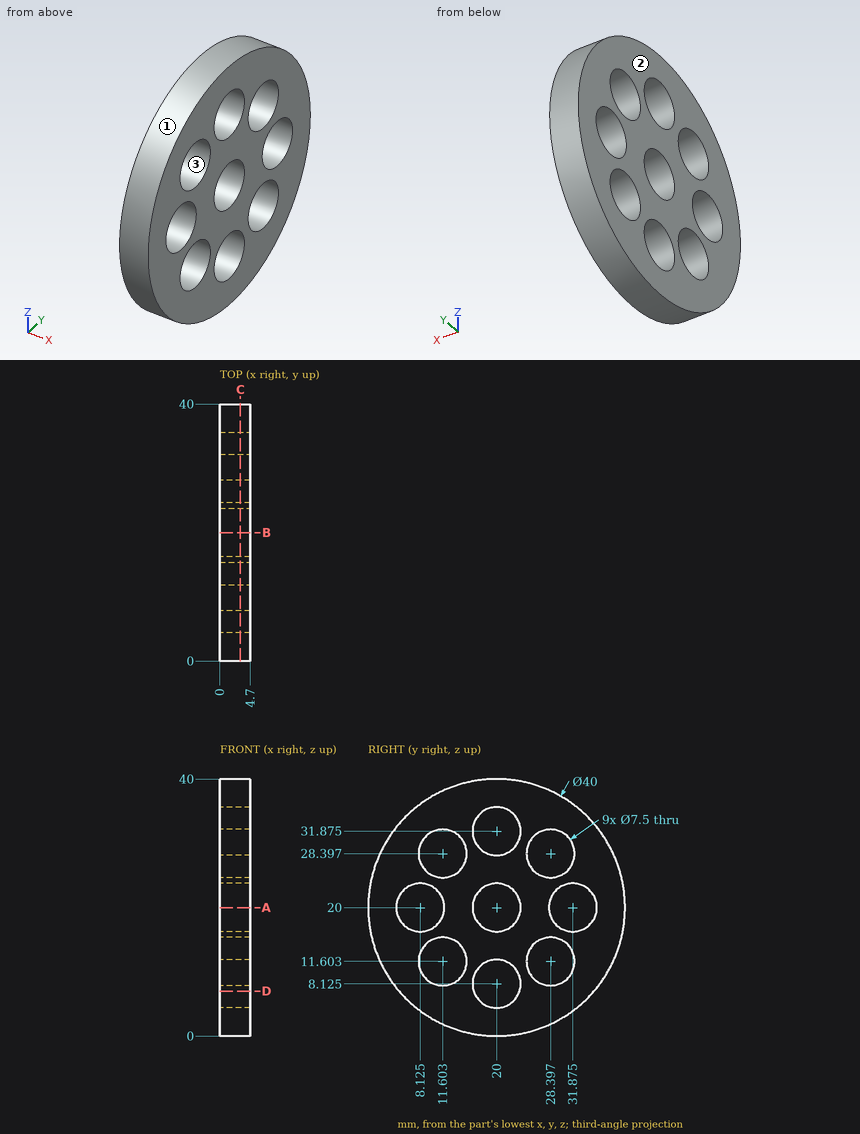
Input: dimensioned drawing with shaded views. Units: mm. Origin: part minimum x, y, z. Give positions to 0.01 mm unless a question says otherwise; leave off trailing zeros. Write each loop counter-clockwise with the first axis right and the second up, starting at its lowest first coordinate (ties: lowest second). Pieces come first, ordered by that corner, then holes. Notation, with made-up numbers: (-13.5, -23) - (9.5, -23) arc R17 cw to (9.5, -2) - close; hole circle Ø9 at (17.5, 7.25). An arc over 180 degrees is marked (long way). Write item = value, one per line. Start each with the question number.
1) Pin query (flat end, axial travel): pin 1 (1 mm diameter, centred on x = 1, y = 6, fed in from -Z); pin 2 (2 mm diameter, centred on x = 2, z = 27.5, fed in from -Y). Return the tip coordinate at first contact, or that it passes through.
2) Cut plane D-D (z = 7). Return loops of the section in (x, y), and give its area (3 significant figures).
3) Cut plane A-A (z = 20). Return loops of the section in (x, y) (3 decimals).
4) Cut plane C-C (x = 3.2). Give the number of separate pieces and of enclosed holes in the cut face, and give its area (3 significant figures).
5) Draft query along Y for the marked faces 1, 2 and 3. Return one class per face: pulls with the +Y half, pulls with the -Y half, needs draft (parallel to the pull), parting line crosses it, or undercut.
6) Material intervals for L1, parallel to Z at x = 2.1, y = 20 (3 decimals); L2, parallel to Z at x = 2.7, y = 22; L3, parallel to Y at x = 0.25, z = 28, sorted ascending. Write a range as [from, to].
Answers follow:
q1.pin_1 = 5.24
q1.pin_2 = 1.09
q2.outline = (0, 4.8) - (4.7, 4.8) - (4.7, 16.42) - (0, 16.42) - close; (0, 23.58) - (4.7, 23.58) - (4.7, 35.2) - (0, 35.2) - close
q2.area = 109 mm^2
q3.outline = (0, 0) - (4.7, 0) - (4.7, 4.375) - (0, 4.375) - close; (0, 11.875) - (4.7, 11.875) - (4.7, 16.25) - (0, 16.25) - close; (0, 23.75) - (4.7, 23.75) - (4.7, 28.125) - (0, 28.125) - close; (0, 35.625) - (4.7, 35.625) - (4.7, 40) - (0, 40) - close
q4.separate_pieces = 1
q4.enclosed_holes = 9
q4.area = 859 mm^2
q5.face_1 = parting line crosses it
q5.face_2 = needs draft
q5.face_3 = undercut
q6.L1 = [0, 4.375], [11.875, 16.25], [23.75, 28.125], [35.625, 40]
q6.L2 = [0.1, 4.95], [11.3, 16.83], [23.17, 28.7], [35.05, 39.9]
q6.L3 = [1.67, 7.87], [15.33, 24.67], [32.13, 38.33]
